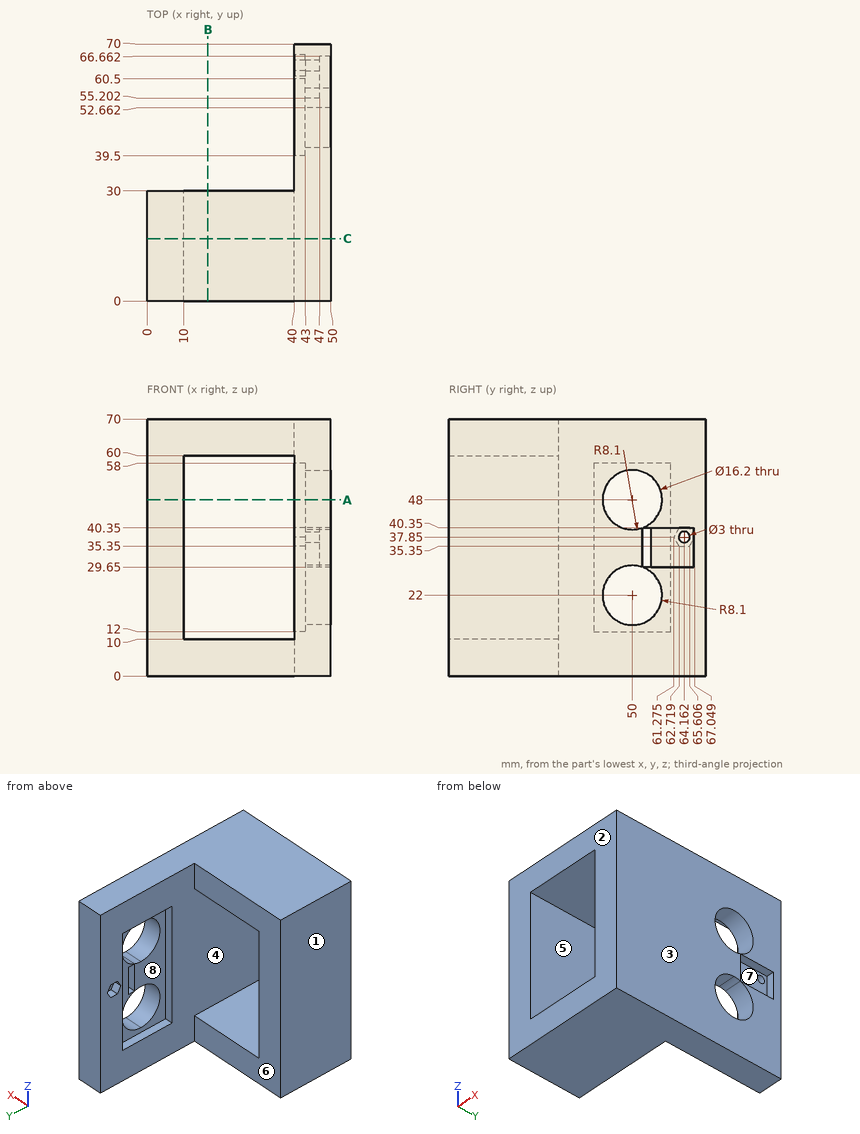
Can you work these out from the drawing? Everything is in mm from the part's minimum corner. A direction names the side the tool comes from. Coordinates: 2 decimals unless noted, no trailing zeros. Write each loop counter-clockwise with the first axis right and the second up, starting at its lowest first coordinate (ties: lowest second). Pieces come first, ordered by that corner, then holes. Notation, with made-up numbers: (-24, -27) -> (-7, -27) arc R31 ccw to (-7, -3) -> close; hole circle Ø7 at (45.5, 5.25). An arc over 180 degrees is marked (long way). Return JSON: item names as keys, results as strings.
(1) Imagine slicing it at A-A, the plane z = 48. Please give me the cut outline in (x, y).
Numbers:
{"outline": "(0, 0) -> (10, 0) -> (10, 30) -> (0, 30) -> close; (40, 0) -> (50, 0) -> (50, 41.9) -> (43, 41.9) -> (43, 39.5) -> (40, 39.5) -> close; (40, 60.5) -> (43, 60.5) -> (43, 58.1) -> (50, 58.1) -> (50, 70) -> (40, 70) -> close"}
(2) Imagine slicing it at B-B, the plane x = 16.5. Please give me the cut outline in (y, z), then the cut area to 3 significant figures.
Numbers:
{"outline": "(0, 0) -> (30, 0) -> (30, 10) -> (0, 10) -> close; (0, 60) -> (30, 60) -> (30, 70) -> (0, 70) -> close", "area": "600 mm2"}
(3) Which directions (+Z, -Z, +X, -X, +Y, -Y) give clear straight access to the entire face, cutting with the end or side of a thin tool? Please do the marked faces 5, 6, 7 and 8.
Numbers:
{"face 5": "+Y, -Y", "face 6": "+Z, -Z, -X, +Y", "face 7": "+X", "face 8": "-X"}
(4) I need wall thicknesses on L1, parallel to Z at x = 46, y = 50; L2, parallel to Y at x = 48.25, z = 48; L3, parallel to Y at x = 45.05, z = 37.85. Which ranges of each line are inside material? Lowest first, please.
Numbers:
{"L1": "z = 0 to 13.9, 30.1 to 39.9, 56.1 to 70", "L2": "y = 0 to 41.9, 58.1 to 70", "L3": "y = 0 to 52.66, 55.2 to 62.66, 65.66 to 70"}
(5) I'm going to push flat-ended pins straight in: pin 1 (12 mm diameter, centred on x = 21, z = 36, fed in from -Y); pin 2 (6 mm diameter, centred on x = 26, z = 7.5, fed in from +Y); pin 3 (21 mm diameter, centred on y = 42, z = 46, fed in from -X); pin 4 (1.5 mm diameter, centred on y = 64, z = 37, fed in from -X). Where does each tip first touch, or does it pass through?
Numbers:
{"pin 1": "passes through", "pin 2": "stops at y = 30", "pin 3": "stops at x = 40", "pin 4": "stops at x = 43"}
(6) Imagine slicing it at C-C, the plane y = 17. Please give me the cut outline in (x, z), then the cut area to 3 significant figures.
Numbers:
{"outline": "(0, 0) -> (50, 0) -> (50, 70) -> (0, 70) -> close; hole (10, 10) -> (40, 10) -> (40, 60) -> (10, 60) -> close", "area": "2,000 mm2"}
(7) We'd pull the mould along X, two halves only. Please class the marked faces 1, 2, 3 and 4: +X half, -X half, draft (parallel to the pull), parting line (faces both ways), or undercut.
Numbers:
{"face 1": "-X half", "face 2": "draft", "face 3": "+X half", "face 4": "undercut"}
